Autodesk Inventor part; units mm, degrees
ref_plane "Work Plane2" through (-104.3093, 2.4643, 13) normal (-0.8618583, -0.5071491, 0) x (-0.5071491, 0.8618583, 0)
ref_plane "Work Plane3" through (-119.6586, 28.5492, 14.2) normal (0, 0, -1) x (-0.5071491, 0.8618583, 0)
ref_plane "Work Plane4" through (-137.8592, 54.6206, 14.2) normal (0, -1, 0) x (-1, 0, 0)
sketch "Sketch1" plane through (0, 0, 0) normal (0, 0, 1) x (1, 0, 0)
  circle A0 centre (0, 0) radius 2.38
  dimension "d0" = 4.76
sketch "Sketch2" plane through (0, 0, 0) normal (0, 1, 0) x (-1, 0, 0)
  line L0 (0, 0) -> (0, 8)
  line L1 (5, 13) -> (100, 13)
  arc A0 (5, 13) -> (0, 8) centre (5, 8) ccw
  point P0 (0, 13)
  dimension "d1" = 13
  dimension "d2" = 100
  dimension "d3" = 5
sweep "Sweep1" add profiles "Sketch1" path "Sketch2"
ref_plane "Work Plane1" through (-5, 0, 13) normal (0, 0, -1) x (-1, 0, 0)
sketch "Sketch3" plane through (-100, 0, 13) normal (-1, 0, 0) x (0, 0, 1)
  circle A0 centre (0, 0) radius 2.38
  point P0 (-13, 0)
sketch "Sketch4" plane through (-5, 0, 13) normal (0, 0, -1) x (-1, 0, 0)
  arc A0 (95, 0) -> (99.3093, 2.4643) centre (95, 5) ccw
  line L0 (95, 2.38) -> (95, -2.38)
  line L1 (-5, -14.1885) -> (-5, 68.471)
  line L2 (-34.856, 0) -> (157.476, 0)
  line L3 (112.2498, 24.4556) -> (99.3093, 2.4643)
  line L4 (130, 54.6206) -> (126.5299, 56.6625)
  point P0 (-5, 0)
  dimension "d6" = 10
  dimension "d11" = 35
  dimension "d44" = 54.6206
  dimension "d45" = 35
sweep "Sweep2" add profiles "Sketch3" path "Sketch4" path curves A0 L3
ref_plane "Work Plane2" through (-104.3093, 2.4643, 13) normal (-0.8618583, -0.5071491, 0) x (-0.5071491, 0.8618583, 0)
sketch "Sketch5" plane through (-117.2498, 24.4556, 13) normal (-0.5071491, 0.8618583, 0) x (0.8618583, 0.5071491, 0)
  circle A0 centre (0, 0) radius 2.38
  point P0 (88.6501, 13)
sketch "Sketch6" plane through (-104.3093, 2.4643, 13) normal (-0.8618583, -0.5071491, 0) x (-0.5071491, 0.8618583, 0)
  line L0 (67.6152, 13) -> (-122.0784, 13)
  line L1 (-122.0784, 13) -> (67.6152, 13)
  line L2 (67.6152, 13) -> (-122.0784, 13)
  line L3 (0, 2.38) -> (0, -2.38)
  arc A0 (27.891, -0.6) -> (25.5161, 0) centre (25.5161, -5) ccw
  line L4 (40.5161, -1.2) -> (30.2659, -1.2)
  arc A1 (27.891, -0.6) -> (30.2659, -1.2) centre (30.2659, 3.8) ccw
  line L5 (25.5161, -5) -> (30.2659, 3.8) construction
  line L6 (25.5161, 2.38) -> (25.5161, -2.38)
  line L7 (0, 2.38) -> (0, -2.38)
  point P0 (-55.0242, 13)
  point P1 (25.5161, 0)
  dimension "d16" = 10
  dimension "d20" = 10
  dimension "d22" = 1.2
  dimension "d23" = 15
sweep "Sweep3" add profiles "Sketch5" path "Sketch6" path curves A0 A1 L4
sketch "Sketch7" plane through (-124.857, 37.3834, 14.2) normal (-0.5071491, 0.8618583, 0) x (0.8618583, 0.5071491, 0)
  circle A0 centre (0, 0) radius 2.38
  point P0 (88.6501, 14.2)
ref_plane "Work Plane3" through (-119.6586, 28.5492, 14.2) normal (0, 0, -1) x (-0.5071491, 0.8618583, 0)
sketch "Sketch8" plane through (-119.6586, 28.5492, 14.2) normal (0, 0, -1) x (-0.5071491, 0.8618583, 0)
  line L0 (-101.837, 116.7703) -> (5.5426, -65.7126)
  line L1 (34.7421, -7.6336) -> (31.7003, -2.4643)
  line L2 (10.2503, 2.38) -> (10.2503, -2.38)
  line L3 (10.2503, 0) -> (27.391, 0)
  arc A0 (31.7003, -2.4643) -> (27.391, 0) centre (27.391, -5) ccw
  point P0 (-85.2901, 88.6501)
  point P1 (37.2779, -11.9428)
  dimension "d27" = 5
  dimension "d28" = 5
  dimension "d41" = 27.0276
  dimension "d42" = 11.9428
sweep "Sweep4" add profiles "Sketch7" path "Sketch8" path curves L3 A0 L1
ref_plane "Work Plane4" through (-137.8592, 54.6206, 14.2) normal (0, -1, 0) x (-1, 0, 0)
sketch "Sketch10" plane through (-143.8571, 54.6206, 14.2) normal (-1, 0, 0) x (0, 0, 1)
  circle A0 centre (0, 0) radius 2.38
  point P0 (-14.2, -54.6206)
sketch "Sketch11" plane through (-137.8592, 54.6206, 14.2) normal (0, -1, 0) x (-1, 0, 0)
  line L0 (5.9979, 2.38) -> (5.9979, -2.38)
  line L1 (-137.8592, -5.856) -> (-137.8592, 18.476)
  line L2 (42.4879, 14.2) -> (-170.6938, 14.2)
  line L3 (10.9979, 15) -> (10.9979, 5)
  line L4 (5.9979, 0) -> (5.9979, 0)
  arc A0 (5.9979, 0) -> (10.9979, 5) centre (5.9979, 5) ccw
  point P0 (-137.8592, 14.2)
  dimension "d33" = 5
  dimension "d34" = 15
  dimension "d43" = 5
sweep "Sweep5" add profiles "Sketch10" path "Sketch11" path curves L4 A0 L3
ref_plane "Work Plane5" through (-5, 0, 13) normal (0, -1, 0) x (-1, 0, 0)
properties part number "100-09" material "Steel"
Geometry check sheet. Reference: the model listing, model coordinates, mm. A direction names the side the tool comes from. Round coordinates to 2 decimals unless told otherwise and drop trailing zeros. Order: outer loops, then holes, each group sorted by start corner. A loop starts at its lowest first (then second) coordinate and runs counter-clockwise, first axis right, second up. Notation, with made-up numbers: M 8,68.5 L 45,68.5 A21 ccw 45,76.5 Z; hole C 7,1.5 d1. An arc over 180 degrees is marked long. Answer in a Markdown table with one row per item. Add a question column.
Item 1: Depth check by flat-ended pin: pin 1 Ø1.4 at (x, y) = (-1, -0.5) entering from -Z; pin 2 Ø5 at (x, z) = (-87, 11.5) entering from +Y; pin 3 Ø6 at (x, z) = (-66, 9) entering from +Y. Enter the tip coordinate at first touch or a pass-through.
Item 2: Draft check along X on faces 1 (the face through (-53.16, 0.71, 15.27)), 2 (the face through (-149, 55, -0.8)), 3 (the face through (-130.776, 43.984, 12.591)). Enter one of: released by +X, released by -X, zero draft, split by the parting line, or undercut.
Item 3: Material ranges on L1, parallel to Z at x = -26.5, y = 1; L2, parallel to Y at x = -100, z = 13; L3, parallel to Y at x = -44.5, z = 13.75, recorded low to high. Write a range as [from, to].
Item 4: Sectioned sample at A-A, the plane z = 5.75. Enter the section's corners in (x, y).
Item 5: Set-up check for faces 4 (the face through (0, 0, 0)), 5 (the face through (-0.516, -2.323, 4.056)): record each of +Z, -Z, +X, -X, +Y, -Y from which the full face is reachable in a straight line by a thin tool's end or side.
Item 6: Sectioned sample at B-B, the plane x = -14. Enter the section's corners in (y, z).
Filled in:
| question | item | result |
|---|---|---|
| 1 | pin 1 | stops at z = 0 |
| 1 | pin 2 | stops at y = 2.38 |
| 1 | pin 3 | stops at y = 2.16 |
| 2 | face 1 | undercut |
| 2 | face 2 | zero draft |
| 2 | face 3 | split by the parting line |
| 3 | L1 | z = [10.84, 15.16] |
| 3 | L2 | y = [-2.38, 2.38] |
| 3 | L3 | y = [-2.26, 2.26] |
| 4 | outline | C -148.86,54.62 d4.76; C 0,0 d4.76 |
| 5 | face 4 | -Z, +X, -X, +Y, -Y |
| 5 | face 5 | -Z |
| 6 | outline | C 0,13 d4.76 |
